```python
from build123d import *

# Parameters (mm, degrees)
SKETCH_1_W          = 15
SKETCH_1_H          = 15
SKETCH_1_W_2        = 13
SKETCH_1_H_2        = 13
EXTRUDE_1_DEPTH     = 100
SKETCH_2_R          = 1.6
CUT_EXTRUDE_1_DEPTH = 103.225241501
SKETCH_3_R          = 1.6
CUT_EXTRUDE_2_DEPTH = 103.225241501


with BuildPart() as part:
    # 草图1 → 拉伸-薄壁1 (new body)
    with BuildSketch(Plane.XY):
        with Locations((7.5, -7.5)):
            Rectangle(SKETCH_1_W, SKETCH_1_H)
        with Locations((7.5, -7.5)):
            Rectangle(SKETCH_1_W_2, SKETCH_1_H_2, mode=Mode.SUBTRACT)
    extrude(amount=EXTRUDE_1_DEPTH)

    # 草图2 → 切除-拉伸1 (cut, through all)
    with BuildSketch(Plane(origin=(15, 0, 0), x_dir=(0, 0, -1), z_dir=(1, 0, 0))):
        with Locations((-75, -3.75)):
            Circle(SKETCH_2_R)
        with Locations((-75, -11.25)):
            Circle(SKETCH_2_R)
        with Locations((-65, -11.25)):
            Circle(SKETCH_2_R)
        with Locations((-65, -3.75)):
            Circle(SKETCH_2_R)
        with Locations((-25, -3.75)):
            Circle(SKETCH_2_R)
        with Locations((-25, -11.25)):
            Circle(SKETCH_2_R)
        with Locations((-35, -11.25)):
            Circle(SKETCH_2_R)
        with Locations((-35, -3.75)):
            Circle(SKETCH_2_R)
    extrude(amount=-CUT_EXTRUDE_1_DEPTH, mode=Mode.SUBTRACT)

    # 草图3 → 切除-拉伸2 (cut, through all)
    with BuildSketch(Plane(origin=(0, 0, 0), x_dir=(1, 0, 0), z_dir=(0, 1, 0))):
        with Locations(Location((3.75, -5, 0), (0, 0, 270))):
            Circle(SKETCH_3_R)
        with Locations(Location((11.25, -5, 0), (0, 0, 90))):
            Circle(SKETCH_3_R)
        with Locations(Location((11.25, -15, 0), (0, 0, 270))):
            Circle(SKETCH_3_R)
        with Locations(Location((3.75, -15, 0), (0, 0, 90))):
            Circle(SKETCH_3_R)
        with Locations(Location((3.75, -45, 0), (0, 0, 270))):
            Circle(SKETCH_3_R)
        with Locations(Location((11.25, -45, 0), (0, 0, 90))):
            Circle(SKETCH_3_R)
        with Locations(Location((11.25, -55, 0), (0, 0, 270))):
            Circle(SKETCH_3_R)
        with Locations(Location((3.75, -55, 0), (0, 0, 90))):
            Circle(SKETCH_3_R)
        with Locations(Location((3.75, -85, 0), (0, 0, 270))):
            Circle(SKETCH_3_R)
        with Locations(Location((11.25, -85, 0), (0, 0, 90))):
            Circle(SKETCH_3_R)
        with Locations(Location((11.25, -95, 0), (0, 0, 270))):
            Circle(SKETCH_3_R)
        with Locations(Location((3.75, -95, 0), (0, 0, 90))):
            Circle(SKETCH_3_R)
    extrude(amount=-CUT_EXTRUDE_2_DEPTH, mode=Mode.SUBTRACT)


solid = part.part
```
Work out the finished part from the listing and answer in its coordinate system (mm). A direction names the side the tool comes from. Give positions to 0.01 mm unless a question says otherwise; leave off trailing zeros. Loops run counter-clockwise (first coordinate to the right, second up) from the corner with the lowest first, then second, coordinate; pieces in that order, holes last. Notation, with made-up numbers: (77.25, 46) - (118.25, 46) arc R16 ccw to (118.25, 69) - close; hole circle Ø5 at (-26.5, 65.5). An arc over 180 degrees is marked (long way). One line per question, with ' | ' between items.
(1) The part is cut by section C-C (z = 85). Write down the section's boundary in (x, y).
Recorded:
outline: (0, -15) - (2.15, -15) - (2.15, -14) - (1, -14) - (1, -1) - (2.15, -1) - (2.15, 0) - (0, 0) - close; (5.35, -15) - (9.65, -15) - (9.65, -14) - (5.35, -14) - close; (5.35, -1) - (9.65, -1) - (9.65, 0) - (5.35, 0) - close; (12.85, -15) - (15, -15) - (15, 0) - (12.85, 0) - (12.85, -1) - (14, -1) - (14, -14) - (12.85, -14) - close
(2) The mould has two halves that part along Y. Classify faces 1 (the face through (7, 0, 49)), 2 (the face through (14.51, -11.86, 63.52)), 3 (the face through (11.2, -14.5, 86.6)): +Y half, -Y half, draft (parallel to the pull), parting line (faces both ways), or undercut.
Recorded:
face 1: +Y half | face 2: undercut | face 3: draft
(3) The part is cut by section B-B (x = 7.5). Write down the section's boundary in (y, z).
Recorded:
outline: (-15, 0) - (-14, 0) - (-14, 100) - (-15, 100) - close; (-1, 0) - (0, 0) - (0, 100) - (-1, 100) - close
(4) The part is cut by section A-A (z = 48.5). Write down the section's boundary in (x, y).
Recorded:
outline: (0, -15) - (15, -15) - (15, 0) - (0, 0) - close; hole (1, -14) - (14, -14) - (14, -1) - (1, -1) - close
(5) The part is cut by section D-D (y = -11.25). Count the separate pieces of the cut face and the enclosed holes in it, then the cut area to 3 significant figures.
Recorded:
separate pieces: 10 | enclosed holes: 0 | area: 174 mm²
(6) A tool of negligible diameter and unlimited length cuts with its end or side. For faces 4 (the face through (7, -14, 49)), 5 (the face through (15, -8, 49)), from which of +Z, -Z, +X, -X, +Y, -Y can it reach the whole face along a straight path? Write none if from no direction.
Recorded:
face 4: +Z, -Z | face 5: +Z, -Z, +X, +Y, -Y
(7) Straight lines are drawn through the part: probe 1 along Y at (x, z) = (14.3, 25); probe 2 along X at (y, z) = (-0.5, 85); probe 3 along X at (y, z) = (-9.5, 15.5). For each, find the intervals that lie inside material, in ascending order.
Recorded:
probe 1: y = -15 to -12.85, -9.65 to -5.35, -2.15 to 0 | probe 2: x = 0 to 2.15, 5.35 to 9.65, 12.85 to 15 | probe 3: x = 0 to 1, 14 to 15
